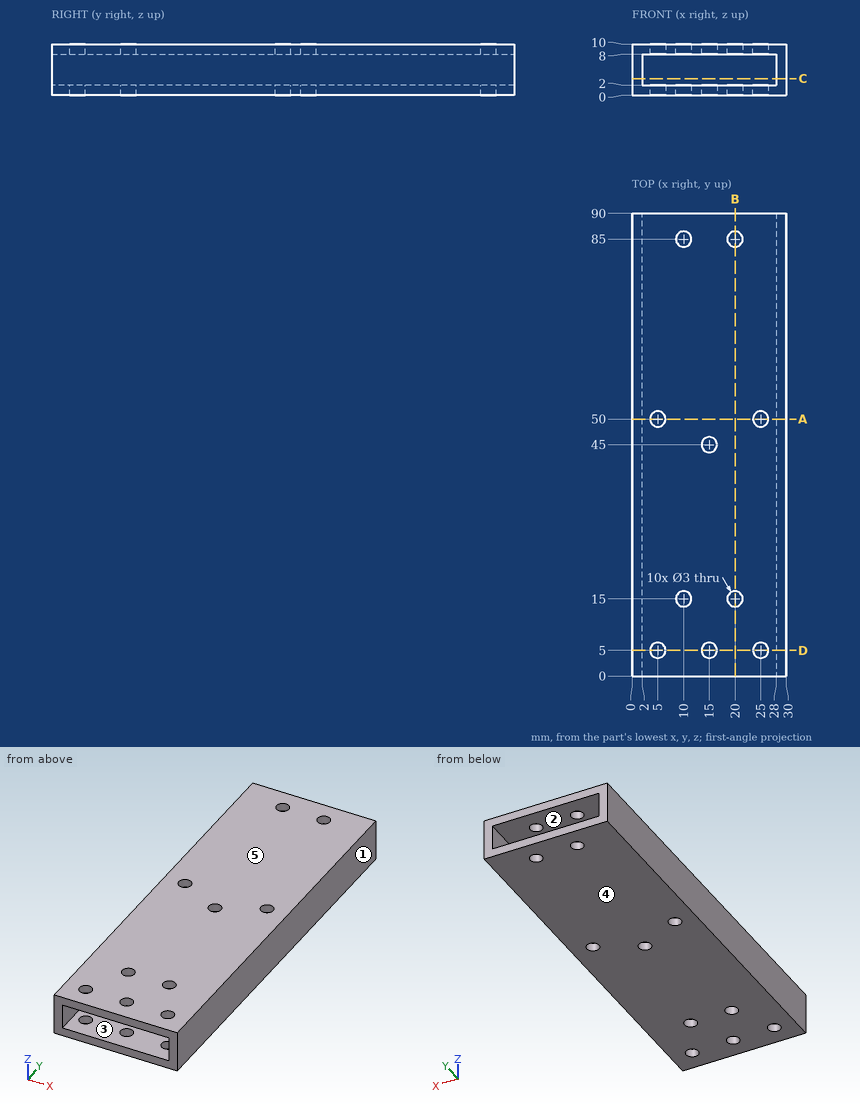
Can you work these out from the drawing? Everything is in mm from the part's minimum corner. A direction names the side the tool comes from. Give positions to 0.01 mm unless a question says otherwise; leave off trailing zeros. Loops run counter-clockwise (first coordinate to the right, second up) from the corner with the lowest first, then second, coordinate; pieces in that order, holes last. Notation, with made-up numbers: M 16,62 L 49,62 A8 ccw 49,67 Z; hole C 30,-29.5 d3. An arc over 180 degrees is marked long. Use CSV: the item, a comma, the result in double quotes. Start each with the question number.
1. Imagine slicing it at D-D, the plane y = 5. Count the separate pieces of the cut face and the enclosed holes in it, plus the area to 3 significant figures.
2. If we mould it in two halves opening along Z, with no side actions, what happens to the marked faces 3, 4 and 5? For each: released by +Z, released by -Z, zero draft, split by the parting line, or undercut.
3. Imagine slicing it at B-B, the plane x = 20. Write out the boundary of the cut face in (y, z), plus the area to 3 significant figures.
4. On a 3-axis mill with a long thin cutter (end or side, diameter ignored), from which of +Z, -Z, +X, -X, +Y, -Y can I reach the whole of each face in a straight line? I mean the marked faces 1 and 2. Say none if no direction works.
5. Imagine slicing it at A-A, the plane y = 50. Write out the boundary of the cut face in (x, z).
6. If I drill on L1, parallel to Y at x = 15, z = 9.2; L2, parallel to Y at x = 20, z = 9.3; L3, parallel to X at y = 85, z = 0.9, over which ranges is the centre line in solid material (lowest first)?
7. For P1, Ø3, axis at y = 47.5, z = 6.5, coming from the -X side; P2, Ø3, axis at x = 18, z = 6, coming from the +Y side, each with a flat end and sliding along its axis, tell me the tip position at first contact or that it passes through.
8. Imagine slicing it at C-C, the plane z = 3.25. Write out the boundary of the cut face in (x, y).
Response values:
1,separate pieces,"6"
1,enclosed holes,"0"
1,area,"108 mm^2"
2,face 3,"undercut"
2,face 4,"released by -Z"
2,face 5,"released by +Z"
3,outline,"M 0,0 L 13.5,0 L 13.5,2 L 0,2 Z; M 0,8 L 13.5,8 L 13.5,10 L 0,10 Z; M 16.5,0 L 83.5,0 L 83.5,2 L 16.5,2 Z; M 16.5,8 L 83.5,8 L 83.5,10 L 16.5,10 Z; M 86.5,0 L 90,0 L 90,2 L 86.5,2 Z; M 86.5,8 L 90,8 L 90,10 L 86.5,10 Z"
3,area,"336 mm^2"
4,face 1,"+Z, -Z, +X, +Y, -Y"
4,face 2,"+Y, -Y"
5,outline,"M 0,0 L 3.5,0 L 3.5,2 L 2,2 L 2,8 L 3.5,8 L 3.5,10 L 0,10 Z; M 6.5,0 L 23.5,0 L 23.5,2 L 6.5,2 Z; M 6.5,8 L 23.5,8 L 23.5,10 L 6.5,10 Z; M 26.5,0 L 30,0 L 30,10 L 26.5,10 L 26.5,8 L 28,8 L 28,2 L 26.5,2 Z"
6,L1,"0 to 3.5, 6.5 to 43.5, 46.5 to 90"
6,L2,"0 to 13.5, 16.5 to 83.5, 86.5 to 90"
6,L3,"0 to 8.5, 11.5 to 18.5, 21.5 to 30"
7,P1,"x = 0"
7,P2,"through"
8,outline,"M 0,0 L 2,0 L 2,90 L 0,90 Z; M 28,0 L 30,0 L 30,90 L 28,90 Z"
